from build123d import *

# Parameters (mm, degrees)
SKETCH002_W     = 24.115805
SKETCH002_H     = 45
PAD001_DEPTH    = 8
POCKET001_DEPTH = 45.001
SKETCH004_W     = 9.473238
SKETCH004_H     = 26.16662
SKETCH004_W_2   = 10.488205
SKETCH004_H_2   = 27.344377
POCKET002_DEPTH = 23.073659
SKETCH005_R     = 2.6
POCKET003_DEPTH = 15.501
CHAMFER_SIZE    = 2
SKETCH007_W     = 5.2
SKETCH007_H     = 7
POCKET004_DEPTH = 16.5
FILLET_R        = 0.5


with BuildPart() as part:
    # Sketch002 → Pad001 (new body, symmetric)
    with BuildSketch(Plane.XZ):
        with Locations((12.214756, 0)):
            Rectangle(SKETCH002_W, SKETCH002_H)
    extrude(amount=PAD001_DEPTH, both=True)

    # Sketch003 (on Face1 of Pad001) → Pocket001 (cut, through all)
    with BuildSketch(Plane(origin=(0, 0, 22.5), x_dir=(-1, 0, 0), z_dir=(0, 0, 1))):
        Polygon((-1.2, 7.5), (-1.2, -7.5), (-11.2, -5), (-26.098127, -5), (-26.098127, -10.333512), (0.566555, -10.333512), (0.566555, 8.419309), (-11.2, 8.419309), (-11.2, 5), align=None)
    extrude(amount=-POCKET001_DEPTH, mode=Mode.SUBTRACT)

    # Sketch004 (on Face8 of Pocket001) → Pocket002 (cut, through all)
    with BuildSketch(Plane(origin=(24.272659, 0, 0), x_dir=(0, 0, 1), z_dir=(1, 0, 0))):
        with Locations((-18.054942, -4.322038)):
            Rectangle(SKETCH004_W, SKETCH004_H)
        with Locations((18.562425, -4.910916)):
            Rectangle(SKETCH004_W_2, SKETCH004_H_2)
    extrude(amount=-POCKET002_DEPTH, mode=Mode.SUBTRACT)

    # Sketch005 (on Face6 of Pocket002) → Pocket003 (cut, through all)
    with BuildSketch(Plane.XZ.offset(8)):
        with Locations((21.316544, 0)):
            Circle(SKETCH005_R)
    extrude(amount=-POCKET003_DEPTH, mode=Mode.SUBTRACT)

    # Chamfer
    chamfer_edges = [part.edges().sort_by_distance(p)[0] for p in [
        (17.73633, 5, -13.318323),
        (17.73633, 5, 13.318323),
    ]]
    chamfer(chamfer_edges, length=CHAMFER_SIZE)

    # Sketch007 (on Face7 of Chamfer) → Pocket004 (cut)
    with BuildSketch(Plane(origin=(0, 0, -13.318323), x_dir=(1, 0, 0), z_dir=(0, 0, -1))):
        with Locations((3.8, 0)):
            Rectangle(SKETCH007_W, SKETCH007_H)
    extrude(amount=-POCKET004_DEPTH, mode=Mode.SUBTRACT)

    # Fillet
    fillet_edges = [part.edges().sort_by_distance(p)[0] for p in [
        (1.2, -7.5, 0),
        (1.2, 7.5, 0),
        (11.2, -5, 0),
    ]]
    fillet(fillet_edges, radius=FILLET_R)


solid = part.part
Check sheet for the modelled part. Datum: model origin and axes. Units: mm. A direction names the side the tool comes from. Give positions to 0.01 mm unless a question says otherwise; leave off trailing zeros. Loops run counter-clockwise (first coordinate to the right, second up) from the corner with the lowest first, then second, coordinate; pieces in that order, holes last. Notation, with made-up numbers: M 28.5,-4.75 L 48.5,-4.75 A15 ccw 48.5,22.25 Z; hole C 18.5,23.5 d6. An arc over 180 degrees is marked long. Answer as a JSON object with one key per item and string values. Group by question number.
Q1. Access from +Z, -Z, +X, -X, +Y, -Y to the whole of each face (thin tool, end or side, straight path). Record for faces 4 (the flat face through (19.28, 4.24, 12.08)), 5 (the flat face through (4, 0, 3.182)), 6 (the flat face through (19.28, 4.24, -12.08)), 7 (the flat face through (6.261, -6.235, 0.186)), 8 (the flat face through (18, 5, 0)).
Q2. Cross-section at A-A on y = -2. Record the cut outline in (x, z).
Q3. Go/stop test with flat-tipped pins: P1, Ø2, axis at y = -1, z = -7, coming from the -X side; P2, Ø2.5, axis at x = 3, z = -2, coming from the -Y side; P3, Ø4, axis at x = 4, y = -0.5, coming from the -Z side; P4, Ø4, axis at x = 21.32, z = 0, coming from the +Y side. Record where each tip stops, or that it passes through.
Q4. Cross-section at B-B on z = -7.5. Record the cut outline in (x, y).
Q5. Cross-section at C-C on z = 0. Record the cut outline in (x, y).
Q6. Cross-section at D-D on x = 20.5. Record the cut outline in (y, z), then the cut area to 3 significant figures.
Q7. Release check for a two-part mould opening along X. For faces 1 (the flat face through (1.2, 0, 6)), 2 (the flat face through (11.2, -7, 0)), 3 (the flat face through (18, -8, 0)) record: released by +X, released by -X, zero draft, split by the parting line, or undercut.
Q8. Material ranges on line 1 along Y through (x, z) = (19, -1.25); line 2 along X through (y, z) = (-1.75, -3.5); line 3 along Y through (x, z) = (3.75, -0.5), recorded low to high. Write a range as [from, to].
Evaluation:
{
 "1": {"face 4": "+Z, +X, +Y", "face 5": "-Z, -X", "face 6": "-Z, +X, +Y", "face 7": "+Z, -Z, -Y", "face 8": "+Z, -Z, +X, +Y"},
 "2": {"outline": "M 1.2,3.18 L 6.4,3.18 L 6.4,-13.32 L 24.27,-13.32 L 24.27,13.32 L 1.2,13.32 Z; hole C 21.32,0 d5.2"},
 "3": {"P1": "stops at x = 6.4", "P2": "stops at y = -7.36", "P3": "stops at z = 3.18", "P4": "passes through"},
 "4": {"outline": "M 1.2,-6.86 A0.5 ccw 1.82,-7.34 L 10.58,-5.16 A0.5 cw 11.2,-5.64 L 11.2,-8 L 24.27,-8 L 24.27,5 L 11.2,5 L 1.82,7.34 A0.5 ccw 1.2,6.86 L 1.2,3.5 L 6.4,3.5 L 6.4,-3.5 L 1.2,-3.5 Z"},
 "5": {"outline": "M 1.2,-6.86 A0.5 ccw 1.82,-7.34 L 10.58,-5.16 A0.5 cw 11.2,-5.64 L 11.2,-8 L 18.72,-8 L 18.72,5 L 11.2,5 L 1.82,7.34 A0.5 ccw 1.2,6.86 L 1.2,3.5 L 6.4,3.5 L 6.4,-3.5 L 1.2,-3.5 Z; M 23.92,-8 L 24.27,-8 L 24.27,5 L 23.92,5 Z"},
 "6": {"outline": "M -8,-13.32 L 3,-13.32 L 5,-11.32 L 5,-2.47 L -8,-2.47 Z; M -8,2.47 L 5,2.47 L 5,11.32 L 3,13.32 L -8,13.32 Z", "area": "278 mm2"},
 "7": {"face 1": "released by -X", "face 2": "undercut", "face 3": "zero draft"},
 "8": {"line 1": "y = [-8, 5]", "line 2": "x = [6.4, 24.27]", "line 3": "y = [-6.86, -3.5], [3.5, 6.86]"}
}
